from build123d import *

# Parameters (mm, degrees)
CUT_EXTRUDE_1_DEPTH = 2.2


with BuildPart() as part:
    # Sketch 1 → Revolve 1 (revolve)
    with BuildSketch(Plane.XY, mode=Mode.PRIVATE) as revolve_1_sk:
        with BuildLine():
            Line((0, 2), (-11.8, 2))
            ThreePointArc((-11.8, 2), (-11.941421356, 2.058578644), (-12, 2.2))
            Line((-12, 2.2), (-12, 3.8))
            ThreePointArc((-12, 3.8), (-13.264955669, 3.101612484), (-14.2, 2))
            Line((-14.2, 2), (-14.2, 0))
            Line((-14.2, 0), (0, 0))
            Line((0, 0), (0, 2))
        make_face()
    revolve(revolve_1_sk.sketch.rotate(Axis((-14.2, 0, 0), (1, 0, 0)), 90), axis=Axis((-14.2, 0, 0), (1, 0, 0)))

    # Sketch 2 → Cut-Extrude 1 (cut)
    with BuildSketch(Plane.ZY.offset(14.2)):
        Polygon((0, 1.443375673), (-1.25, 0.721687836), (-1.25, -0.721687836), (0, -1.443375673), (1.25, -0.721687836), (1.25, 0.721687836), align=None)
    extrude(amount=-CUT_EXTRUDE_1_DEPTH, mode=Mode.SUBTRACT)

    # Sketch 6 → Revolve 2 (revolve)
    with BuildSketch(Plane.XY):
        Polygon((-12.9, 1.443375673), (-12, 0), (-11.63, 0), (-11.63, 1.443375673), align=None)
    revolve(axis=Axis((-14.2, 0, 0), (1, 0, 0)))

    # Sketch 7 → Cut-Revolve 5 (revolve, cut)
    with BuildSketch(Plane.XY):
        Polygon((-14.2, 1.443375673), (-13.83, 0), (-14.2, 0), align=None)
    revolve(axis=Axis((-14.2, 0, 0), (1, 0, 0)), mode=Mode.SUBTRACT)

    # Sketch 4 → Cut-Revolve 1 (revolve, cut)
    with BuildSketch(Plane.XY, mode=Mode.PRIVATE) as cut_revolve_1_sk:
        Polygon((-0.35, 2), (0, 1.393782217), (0.35, 2), align=None)
    revolve(cut_revolve_1_sk.sketch.rotate(Axis((-0.35, 0, 0), (1, 0, 0)), 90), axis=Axis((-0.35, 0, 0), (1, 0, 0)), mode=Mode.SUBTRACT)


solid = part.part
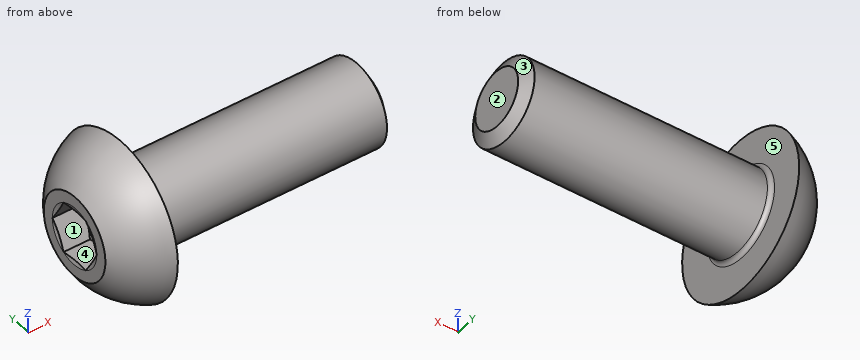
The model under review builds one solid part; all positions refer to its coordinate system, in mm. Face numbers are marked on the shaded views. A direction names the side the tool comes from. Coordinates: 2 decimals unless noted, no trailing zeros. Write each loop counter-clockwise with the first axis right and the second up, starting at its lowest first coordinate (ties: lowest second). Pieces come first, ordered by that corner, then holes. Notation, with made-up numbers: (46, 42) - (96, 42) arc R31 cw to (96, 77) - close; hole circle Ø10 at (88.5, -17.75). An arc over 180 degrees is marked (long way). Answer as CSV lines item,"result".
(1) Clearance check with flat-ended pins moving along their axes: pin 1 Ø1.1 at (x, y) = (-14, 0) entering from -Z; pin 2 Ø2 at (x, y) = (-6.5, -0.5) entering from +Z; pin 3 Ø0.7 at (x, y) = (-13.5, 0) entering from +Z. State where each tip first meets the part, or that it passes through.
Data:
pin 1,"stops at z = -2.94"
pin 2,"stops at z = 2"
pin 3,"stops at z = 3.19"
(2) For line 1 along Y through (x, z) = (-1.5, 0); line 2 along Y through (x, z) = (-3.75, 1.75); line 3 along X through (y, z) = (-2.5, 0), list the stretches that pass through material, from the lowest coordinate up. Write a range as [from, to].
Data:
line 1,"y = [-2, 2]"
line 2,"y = [-0.97, 0.97]"
line 3,"x = [-13.86, -12]"
(3) We need section A-A (x = -8). Give the boundary of the cut face in (y, z).
Data:
outline,"circle Ø4 at (0, 0)"
(4) Mouldability with a two-part tool opening along Z and no side actions: class the marked faces 1, 2 and 3 as pulls with the +Z half, pulls with the -Z half, needs draft (parallel to the pull), parting line crosses it, or undercut.
Data:
face 1,"undercut"
face 2,"needs draft"
face 3,"parting line crosses it"
(5) We need section C-C (z = 3). Give the boundary of the cut face in (x, y), plus the area to 3 significant figures.
Data:
outline,"(-12, -2.33) - (-12, 2.33) arc R2.66 ccw to start"
area,"4.59 mm2"
(6) We need section B-B (z = -2.75). Give the boundary of the cut face in (x, y), plus the area to 3 significant figures.
Data:
outline,"(-12, -2.62) - (-12, 2.62) arc R2.92 ccw to start"
area,"6.17 mm2"
(7) Tool access review of the marked faces 4 and 5: name each direction out of +Z, -Z, +X, -X, +Y, -Y from which nothing blocks a thin tool from reaching the whole face with its end or side.
Data:
face 4,"-X"
face 5,"+X"
